```python
from build123d import *

# Parameters (mm, degrees)
SKETCH2_W           = 30
SKETCH2_H           = 30
BOSS_EXTRUDE1_DEPTH = 15
FILLET1_R           = 4
CHAMFER1_SIZE       = 3
FILLET2_R           = 1
SKETCH4_R           = 10
BOSS_EXTRUDE2_DEPTH = 5
FILLET3_R           = 5
SKETCH6_W           = 5
SKETCH6_H           = 15
BOSS_EXTRUDE3_DEPTH = 20
CHAMFER2_SIZE       = 2
SKETCH7_R           = 5
CUT_EXTRUDE1_DEPTH  = 10
SKETCH8_R           = 0.75
BOSS_EXTRUDE4_DEPTH = 40
CIRPATTERN1_COUNT   = 8
SKETCH10_R          = 5
CUT_EXTRUDE3_DEPTH  = 10
CUT_EXTRUDE4_DEPTH  = 1
LPATTERN1_COUNT     = 2
LPATTERN1_PITCH     = 8
LPATTERN1_COL_COUNT = 2
LPATTERN1_COL_PITCH = 8


# Some blends are built 0.0001 mm under size
with BuildPart() as part:
    # Sketch2 → Boss-Extrude1 (new, symmetric)
    with BuildSketch(Plane.XY):
        Rectangle(SKETCH2_W, SKETCH2_H)
    extrude(amount=BOSS_EXTRUDE1_DEPTH, both=True)

    # Sketch3 → Revolve1 (revolve)
    with BuildSketch(Plane(origin=(0, 0, 0), x_dir=(0, 0, -1), z_dir=(1, 0, 0))):
        Polygon((-15, 0), (-15, 9), (-52, 9), (-52, 15), (-55, 15), (-55, 0), align=None)
    revolve(axis=Axis((0, 0, 15), (0, 0, 1)))

    # Fillet1
    fillet1_edges = [part.edges().sort_by_distance(p)[0] for p in [
        (15, -15, 0),
        (-15, -15, 0),
        (-15, 15, 0),
        (15, 15, 0),
    ]]
    fillet(fillet1_edges, radius=FILLET1_R)

    # Chamfer1
    # the kernel refuses this chamfer: 3 mm, written as the material it takes off along each edge
    with BuildSketch(Plane(origin=(18.715048964, 15, 15), x_dir=(0, -0.9996219169112969, 0.02749587661058621), z_dir=(-1, 0, 0))) as chamfer1_piece_1:
        Polygon((CHAMFER1_SIZE * 0.999621916911, -CHAMFER1_SIZE * 0.0274958766106), (-CHAMFER1_SIZE * 0.0274958766106, -CHAMFER1_SIZE * 0.999621916911), (0, 0), align=None)
    extrude(amount=37.430097928, mode=Mode.SUBTRACT)

    # Fillet2
    fillet2_edges = [part.edges().sort_by_distance(p)[0] for p in [
        (-13.828427125, 13.828427125, -15),
        (0, 15, -15),
        (13.828427125, 13.828427125, -15),
        (15, 0, -15),
        (13.828427125, -13.828427125, -15),
        (0, -15, -15),
        (-13.828427125, -13.828427125, -15),
        (-14.968118785, 11.50401717, 15),
        (14.968118785, 11.50401717, 15),
        (15, 0, 15),
        (13.828427125, -13.828427125, 15),
        (0, -15, 15),
        (-13.828427125, -13.828427125, 15),
        (-15, 0, -15),
        (-15, 0, 15),
    ]]
    fillet(fillet2_edges, radius=FILLET2_R)

    # Sketch4 → Boss-Extrude2 (add)
    with BuildSketch(Plane(origin=(0, 0, -15), x_dir=(-1, 0, 0), z_dir=(0, 0, -1))):
        Circle(SKETCH4_R)
    extrude(amount=BOSS_EXTRUDE2_DEPTH)

    # Fillet3
    fillet3_edges = [part.edges().sort_by_distance(p)[0] for p in [
        (10, 0, -20),
    ]]
    fillet(fillet3_edges, radius=FILLET3_R - 0.0001)  # a hair under: the kernel refuses the full size

    # Sketch6 → Boss-Extrude3 (add)
    with BuildSketch(Plane(origin=(0, 0, -15), x_dir=(-1, 0, 0), z_dir=(0, 0, -1))):
        with Locations((-15, 0)):
            Rectangle(SKETCH6_W, SKETCH6_H)
    extrude(amount=-BOSS_EXTRUDE3_DEPTH)

    # Chamfer2
    chamfer2_edges = [part.edges().sort_by_distance(p)[0] for p in [
        (17.5, 7.5, -5),
        (17.5, 0, 5),
        (17.5, -7.5, -5),
    ]]
    chamfer(chamfer2_edges, length=CHAMFER2_SIZE)

    # Sketch7 → Cut-Extrude1 (cut)
    with BuildSketch(Plane.XY.offset(55)):
        Circle(SKETCH7_R)
    extrude(amount=-CUT_EXTRUDE1_DEPTH, mode=Mode.SUBTRACT)

    # Sketch8 → Boss-Extrude4 (add)
    with BuildSketch(Plane.XY.offset(55)):
        with Locations(Location((0, 11, 0), (0, 0, 90))):
            Circle(SKETCH8_R)
    boss_extrude4 = extrude(amount=-BOSS_EXTRUDE4_DEPTH)

    # CirPattern1: Boss-Extrude4 ×8 about axis
    cirpattern1_axis = Axis((0, 0, 0), (0, 0, 1))
    for i in range(1, CIRPATTERN1_COUNT):
        add(boss_extrude4.rotate(cirpattern1_axis, i * 360 / CIRPATTERN1_COUNT))

    # Sketch10 → Cut-Extrude3 (cut)
    with BuildSketch(Plane.ZY.offset(15)):
        Circle(SKETCH10_R)
    extrude(amount=-CUT_EXTRUDE3_DEPTH, mode=Mode.SUBTRACT)

    # Sketch11 → Cut-Extrude4 (cut)
    with BuildSketch(Plane(origin=(0, 15, 0), x_dir=(1, 0, 0), z_dir=(0, 1, 0))):
        with BuildLine():
            Line((-1, -8), (-1, 8))
            ThreePointArc((-1, 8), (0, 9), (1, 8))
            Line((1, 8), (1, -8))
            ThreePointArc((1, -8), (0, -9), (-1, -8))
        make_face()
    cut_extrude4 = extrude(amount=-CUT_EXTRUDE4_DEPTH, mode=Mode.SUBTRACT)

    # LPattern1: Cut-Extrude4 ×2
    with Locations(*[(i * LPATTERN1_PITCH, 0, 0) for i in range(1, LPATTERN1_COUNT)]):
        add(cut_extrude4, mode=Mode.SUBTRACT)

    # LPattern1 col: Cut-Extrude4 ×2
    with Locations(*[(-i * LPATTERN1_COL_PITCH, 0, 0) for i in range(1, LPATTERN1_COL_COUNT)]):
        add(cut_extrude4, mode=Mode.SUBTRACT)


solid = part.part
```
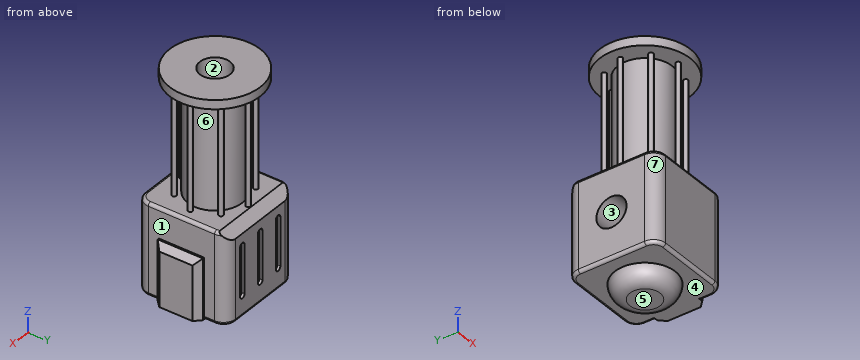
Verification items for the finished model (mm, model axes). Face numbers are marked on the shaded views. A direction names the side the tool comes from. Coordinates: 2 decimals unless noted, no trailing zeros. Put each result on its own line as item: value. Start each with the question number.
1) Tool access check on the marked faces 1, 2, 3 and 4. Record the directions out of +Z, -Z, +X, -X, +Y, -Y that give a thin tool (end or side, any length) a straight path to the whole face; none if there is none.
2) Go/stop test with flat-tipped pins: pin 1 (1 mm diameter, centred on x = -8, z = 3.5, fed in from +Y); pin 2 (5 mm diameter, centred on y = -3, z = 34, fed in from +X); pin 3 (4 mm diameter, centred on x = -8.5, y = -11.5, fed in from -Z). Record where each tip stops, or that it passes through.
3) Cross-section at A-A (z = 26). State how many separate pieces and enclosed holes the cut face has, plus the area to 3 significant figures.
4) Material ranges on L1, parallel to Z at x = 11.5, y = 7; L2, parallel to Z at x = -11, y = 1; L3, parallel to X at y = 14.5, z = -1, recorded low to high.
5) Release check for a two-part mould opening along Z. For the marked faces 5, 6 and 7 record: pulls with the +Z half, pulls with the -Z half, needs draft (parallel to the pull), parting line crosses it, or undercut.
Geometry check:
1. face 1: +Z, +X
1. face 2: +Z
1. face 3: -X
1. face 4: -Z
2. pin 1: stops at y = 14
2. pin 2: stops at x = 11.56
2. pin 3: stops at z = -15
3. separate pieces: 9
3. enclosed holes: 0
3. area: 269 mm^2
4. L1: z = -15 to 15, 52 to 55
4. L2: z = -15 to -4.9, 4.9 to 15, 52 to 55
4. L3: x = -12.94 to -9, -7 to -1, 1 to 7, 9 to 12.94
5. face 5: pulls with the -Z half
5. face 6: undercut
5. face 7: needs draft
